```python
from build123d import *

# Parameters (mm, degrees)
CHAMFER1_SIZE           = 1
CUT_EXTRUDE1_DEPTH      = 45.907070713
CUT_EXTRUDE1_DEPTH_BACK = 45.907070713
SKETCH3_W               = 11.997849067
SKETCH3_H               = 0.999274346
SKETCH3_W_2             = 11.999787666
CUT_EXTRUDE2_DEPTH      = 3


with BuildPart() as part:
    # Sketch2 → Revolve1 (revolve)
    with BuildSketch(Plane.XY, mode=Mode.PRIVATE) as revolve1_sk:
        Polygon((33, 6.35), (-33, 6.35), (-33, 5), (-44, 5), (-44, 0), (44, 0), (44, 5), (33, 5), align=None)
    revolve(revolve1_sk.sketch.rotate(Axis((-44, 0, 0), (1, 0, 0)), 90), axis=Axis((-44, 0, 0), (1, 0, 0)))

    # Chamfer1
    chamfer1_edges = [part.edges().sort_by_distance(p)[0] for p in [
        (44, 0, -5),
        (-44, 0, -5),
    ]]
    chamfer(chamfer1_edges, length=CHAMFER1_SIZE)

    # Sketch3 → Cut-Extrude1 (cut, two sides: drawn at the far end of the back side and taken through both)
    with BuildSketch(Plane.XY.offset(-CUT_EXTRUDE1_DEPTH_BACK)):
        with Locations((5.001075466, 5.850362827)):
            Rectangle(SKETCH3_W, SKETCH3_H)
        with Locations((-24.000665712, 5.850362827)):
            Rectangle(SKETCH3_W_2, SKETCH3_H)
    extrude(amount=CUT_EXTRUDE1_DEPTH + CUT_EXTRUDE1_DEPTH_BACK, mode=Mode.SUBTRACT)

    # Sketch6 → Cut-Extrude2 (cut)
    with BuildSketch(Plane(origin=(0, -6.35, 0), x_dir=(1, 0, 0), z_dir=(0, 1, 0))):
        with BuildLine():
            Line((19.5, 2.5), (-7.500665679, 2.5))
            ThreePointArc((-7.500665679, 2.5), (-9.268432632, 1.767766953), (-10.000665679, 0))
            Line((-10.000665679, 0), (-10.000665679, -0.006446088))
            ThreePointArc((-10.000665679, -0.006446088), (-9.271361564, -1.767141973), (-7.510665679, -2.496446088))
            Line((-7.510665679, -2.496446088), (19.51, -2.496446088))
            ThreePointArc((19.51, -2.496446088), (21.270695885, -1.767141973), (22, -0.006446088))
            Line((22, -0.006446088), (22, 0))
            ThreePointArc((22, 0), (21.267766953, 1.767766953), (19.5, 2.5))
        make_face()
    extrude(amount=CUT_EXTRUDE2_DEPTH, mode=Mode.SUBTRACT)


solid = part.part
```
CAD build for the part. Positions are in the model's coordinates, mm. A direction names the side the tool comes from. Round coordinates to 2 decimals unless told otherwise and drop trailing zeros. Order: outer loops, then holes, each group sorted by start corner. A loop starts at its lowest first (then second) coordinate and runs counter-clockwise, first axis right, second up.
Q1. Slice it at A-A (x = 7). Write the cut outline in (y, z), and give its area (3 significant figures).
Q2. Drop flat-ended pins along their axis: pin 1 (4 mm diameter, centred on x = -23.5, z = -4.5, fed in from -Y); pin 2 (1.1 mm diameter, centred on y = 6, z = -1.5, fed in from +X); pin 3 (3.5 mm diameter, centred on x = 2.5, z = 1.5, fed in from +Y). Give the stop position or say it passes through.
Q3. Slice it at C-C (x = -25). Write the cut outline in (y, z).
Q4. Which spindle directions (+Z, -Z, +X, -X, +Y, -Y) get a long thin tool onto all of the face, cutting with end or side? Do faces 4 (the flat face through (-24, 5.351, 0)), 5 (the cylindrical face through (21, -5, 2)), 6 (the cylindrical face through (38, 0, -5)), 7 (the cylindrical face through (-38, 0, -5)). Say none if no direction does.
Q5. Two-plate mould, pull along X, no slides. Class faces 1 (the flat face through (44, 0, 0)), 2 (the flat face through (-33, 5, 2)), 3 (the cylindrical face through (-9, -5, 2)): pulls with the +X half, pulls with the -X half, needs draft (parallel to the pull), parting line crosses it, or undercut.
Q6. Slice it at D-D (x = 20.5). Write the cut outline in (y, z).
Q7. Wall check: L1, parallel to X at y = 5.5, z = -0.5; L2, parallel to X at y = -4.75, z = -1; L3, parallel to Y at x = 36.5, z = -0.25. Give the ranges that are in metal, low to high.
Q8. Slice it at B-B (y = 0). Write the cut outline in (x, z), and give its area (3 significant figures).
Results below:
1. outline: (-5.84, -2.5) arc R6.35 ccw to (5.35, -3.42) - (5.35, 3.42) arc R6.35 ccw to (-5.84, 2.5) - (-3.35, 2.5) - (-3.35, -2.5) - close
1. area: 108 mm2
2. pin 1: stops at y = -5.84
2. pin 2: stops at x = 33
2. pin 3: stops at y = 5.35
3. outline: (5.35, -3.42) - (5.35, 3.42) arc R6.35 ccw (long way) to start
4. face 4: +Z, -Z, +Y
4. face 5: -Y
4. face 6: +X
4. face 7: -X
5. face 1: pulls with the +X half
5. face 2: pulls with the -X half
5. face 3: undercut
6. outline: (-5.92, -2.29) arc R6.35 ccw (long way) to (-5.92, 2.29) - (-3.35, 2.29) - (-3.35, -2.29) - close
7. L1: x = -33 to -30, -18 to -1, 11 to 33
7. L2: x = -43.15 to -9.79, 21.79 to 43.15
7. L3: y = -4.99 to 4.99
8. outline: (-44, -4) - (-43, -5) - (-33, -5) - (-33, -6.35) - (33, -6.35) - (33, -5) - (43, -5) - (44, -4) - (44, 4) - (43, 5) - (33, 5) - (33, 6.35) - (-33, 6.35) - (-33, 5) - (-43, 5) - (-44, 4) - close
8. area: 1,060 mm2
